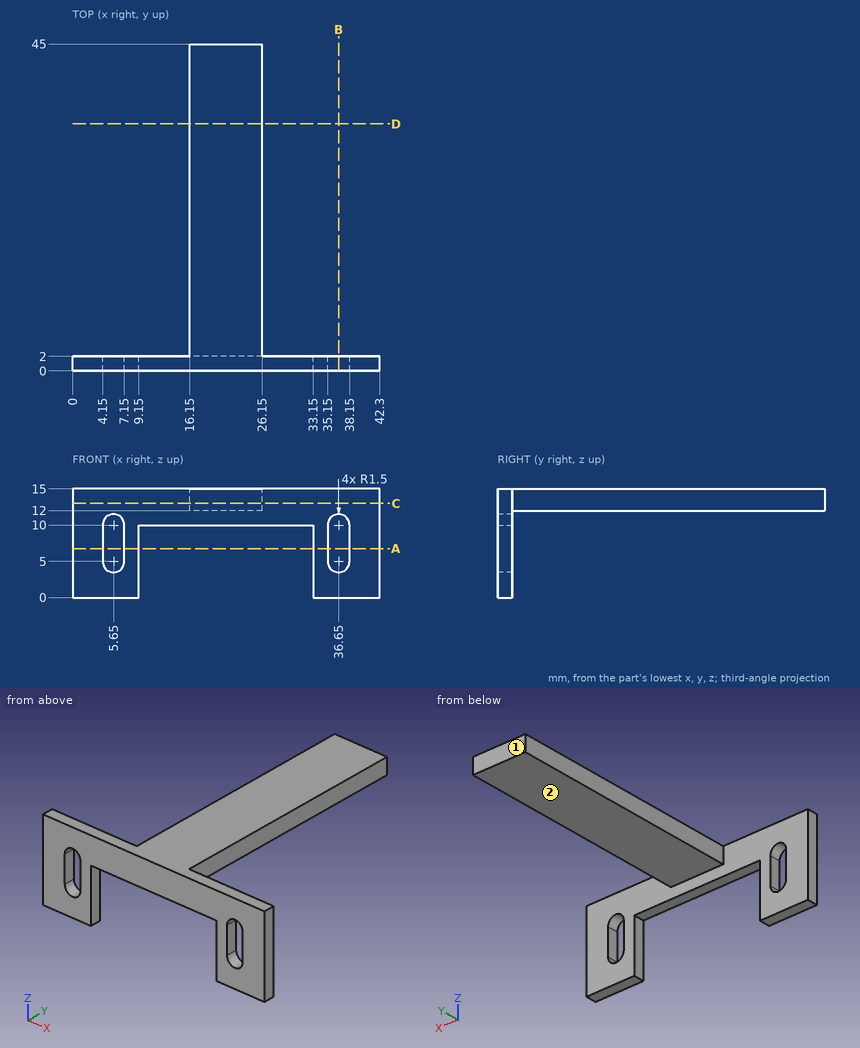
Part print with two shaded views. Sizes in mm from the minimum x, y, z corner. A direction names the side the tool comes from. Coordinates: 2 decimals unless noted, no trailing zeros. Write each loop counter-clockwise with the first axis right and the second up, starting at its lowest first coordinate (ties: lowest second). Pieces come first, ordered by that corner, then holes. Notation, with made-up numbers: (-5.75, 46) - (13.25, 46) arc R25 ccw to (13.25, 69) - close; hole circle Ø9 at (3.5, 57). An arc over 180 degrees is marked (long way). Use a Markdown table: item, result. Add a question column.
Item 1: Band-saw the part on B-B, the plane x = 36.65. Write the cut outline in (y, z), and give its area (3 significant figures).
Item 2: Band-saw the part on C-C, the plane z = 13. Write the cut outline in (x, y).
Item 3: Band-saw the part on A-A, the plane z = 6.75. Write the cut outline in (x, y).
Item 4: Band-saw the part on D-D, the plane y = 34. Write the cut outline in (x, z), and give its area (3 significant figures).
Item 5: Drill centre lines: line 1 along Y through (x, z) = (40, 2); line 2 along Z through (x, y) = (24, 27); line 3 along X through (y, z) = (15, 13). Where is each one in solid material? Low to high.
Item 6: 3-axis set-ups, long thin cutter, end or side, ignore diameter. For the marked faces 1 and 2: which of +Z, -Z, +X, -X, +Y, -Y reach the whole face in a straight line?
Item 7: Drop flat-ended pins along their axis: pin 1 (1.6 mm diameter, centred on x = 24.5, y = 1.5, fed in from -Z); pin 2 (8 mm diameter, centred on y = 11.5, z = 5.5, fed in from +X); pin 3 (10 mm diameter, centred on x = 22, y = 16, fed in from -Z); pin 4 (2.5 mm diameter, centred on y = 14, z = 13, fed in from -X). Give the stop position or say it passes through.
A:
| question | item | result |
|---|---|---|
| 1 | outline | (0, 0) - (2, 0) - (2, 3.5) - (0, 3.5) - close; (0, 11.5) - (2, 11.5) - (2, 15) - (0, 15) - close |
| 1 | area | 14.0 mm² |
| 2 | outline | (0, 0) - (42.3, 0) - (42.3, 2) - (26.15, 2) - (26.15, 45) - (16.15, 45) - (16.15, 2) - (0, 2) - close |
| 3 | outline | (0, 0) - (4.15, 0) - (4.15, 2) - (0, 2) - close; (7.15, 0) - (9.15, 0) - (9.15, 2) - (7.15, 2) - close; (33.15, 0) - (35.15, 0) - (35.15, 2) - (33.15, 2) - close; (38.15, 0) - (42.3, 0) - (42.3, 2) - (38.15, 2) - close |
| 4 | outline | (16.15, 12) - (26.15, 12) - (26.15, 15) - (16.15, 15) - close |
| 4 | area | 30.0 mm² |
| 5 | line 1 | y = 0 to 2 |
| 5 | line 2 | z = 12 to 15 |
| 5 | line 3 | x = 16.15 to 26.15 |
| 6 | face 1 | +Z, -Z, +X, -X, +Y |
| 6 | face 2 | -Z, +X, -X, +Y |
| 7 | pin 1 | stops at z = 10 |
| 7 | pin 2 | passes through |
| 7 | pin 3 | stops at z = 12 |
| 7 | pin 4 | stops at x = 16.15 |
